Read the model definition and answer for the solid it produces. Units are mm, in the model's axes. A direction names the side the tool comes from. Give positions to 0.01 mm unless a question says otherwise; leave off trailing zeros. Order: outer loops, then holes, each group sorted by start corner. A loop starts at its lowest first (then second) coordinate and runs counter-clockwise, first axis right, second up. Notation, with made-up numbers: (26, 66) - (69, 66) arc R9 ccw to (69, 83) - close; hole circle Ø1 at (79, 1.25). An arc over 180 degrees is marked (long way). One line per item, written item: value. Start each with the question number.
```python
from build123d import *

# Parameters (mm, degrees)
F0_R     = 1
F1_DEPTH = 10


with BuildPart() as f1:
    # F0 (on Front) → F1 (new body)
    with BuildSketch(Plane.XZ):
        with BuildLine():
            Line((-1.562834, 8.86327), (-1.345773, 7.63226))
            ThreePointArc((-1.345773, 7.63226), (-2.005848, 7.485925), (-2.650656, 7.282618))
            Line((-2.650656, 7.282618), (-3.078181, 8.457234))
            ThreePointArc((-3.078181, 8.457234), (-3.540527, 8.860187), (-4.094507, 9.123322))
            Line((-4.094507, 9.123322), (-4.356972, 9.000933))
            ThreePointArc((-4.356972, 9.000933), (-4.51149, 8.407419), (-4.5, 7.794229))
            Line((-4.5, 7.794229), (-3.875, 6.711697))
            ThreePointArc((-3.875, 6.711697), (-4.445217, 6.348428), (-4.981604, 5.936844))
            Line((-4.981604, 5.936844), (-5.785088, 6.8944))
            ThreePointArc((-5.785088, 6.8944), (-6.357369, 7.114921), (-6.967938, 7.172715))
            Line((-6.967938, 7.172715), (-7.172715, 6.967938))
            ThreePointArc((-7.172715, 6.967938), (-7.114921, 6.357369), (-6.8944, 5.785088))
            Line((-6.8944, 5.785088), (-5.936844, 4.981604))
            ThreePointArc((-5.936844, 4.981604), (-6.348428, 4.445217), (-6.711697, 3.875))
            Line((-6.711697, 3.875), (-7.794229, 4.5))
            ThreePointArc((-7.794229, 4.5), (-8.407419, 4.51149), (-9.000933, 4.356972))
            Line((-9.000933, 4.356972), (-9.123322, 4.094507))
            ThreePointArc((-9.123322, 4.094507), (-8.860187, 3.540527), (-8.457234, 3.078181))
            Line((-8.457234, 3.078181), (-7.282618, 2.650656))
            ThreePointArc((-7.282618, 2.650656), (-7.485925, 2.005848), (-7.63226, 1.345773))
            Line((-7.63226, 1.345773), (-8.86327, 1.562834))
            ThreePointArc((-8.86327, 1.562834), (-9.44341, 1.363908), (-9.948283, 1.015714))
            Line((-9.948283, 1.015714), (-9.973523, 0.727218))
            ThreePointArc((-9.973523, 0.727218), (-9.536784, 0.296644), (-9, 0))
            Line((-9, 0), (-7.75, 0))
            ThreePointArc((-7.75, 0), (-7.720509, -0.675457), (-7.63226, -1.345773))
            Line((-7.63226, -1.345773), (-8.86327, -1.562834))
            ThreePointArc((-8.86327, -1.562834), (-9.340387, -1.948183), (-9.695722, -2.448054))
            Line((-9.695722, -2.448054), (-9.620769, -2.727784))
            ThreePointArc((-9.620769, -2.727784), (-9.063104, -2.983018), (-8.457234, -3.078181))
            Line((-8.457234, -3.078181), (-7.282618, -2.650656))
            ThreePointArc((-7.282618, -2.650656), (-7.023885, -3.275292), (-6.711697, -3.875))
            Line((-6.711697, -3.875), (-7.794229, -4.5))
            ThreePointArc((-7.794229, -4.5), (-8.110775, -5.025293), (-8.273715, -5.616551))
            Line((-8.273715, -5.616551), (-8.107608, -5.853776))
            ThreePointArc((-8.107608, -5.853776), (-7.496279, -5.902884), (-6.8944, -5.785088))
            Line((-6.8944, -5.785088), (-5.936844, -4.981604))
            ThreePointArc((-5.936844, -4.981604), (-5.480078, -5.480078), (-4.981604, -5.936844))
            Line((-4.981604, -5.936844), (-5.785088, -6.8944))
            ThreePointArc((-5.785088, -6.8944), (-5.902884, -7.496279), (-5.853776, -8.107608))
            Line((-5.853776, -8.107608), (-5.616551, -8.273715))
            ThreePointArc((-5.616551, -8.273715), (-5.025293, -8.110775), (-4.5, -7.794229))
            Line((-4.5, -7.794229), (-3.875, -6.711697))
            ThreePointArc((-3.875, -6.711697), (-3.275292, -7.023885), (-2.650656, -7.282618))
            Line((-2.650656, -7.282618), (-3.078181, -8.457234))
            ThreePointArc((-3.078181, -8.457234), (-2.983018, -9.063104), (-2.727784, -9.620769))
            Line((-2.727784, -9.620769), (-2.448054, -9.695722))
            ThreePointArc((-2.448054, -9.695722), (-1.948183, -9.340387), (-1.562834, -8.86327))
            Line((-1.562834, -8.86327), (-1.345773, -7.63226))
            ThreePointArc((-1.345773, -7.63226), (-0.675457, -7.720509), (0, -7.75))
            Line((0, -7.75), (0, -9))
            ThreePointArc((0, -9), (0.296644, -9.536784), (0.727218, -9.973523))
            Line((0.727218, -9.973523), (1.015714, -9.948283))
            ThreePointArc((1.015714, -9.948283), (1.363908, -9.44341), (1.562834, -8.86327))
            Line((1.562834, -8.86327), (1.345773, -7.63226))
            ThreePointArc((1.345773, -7.63226), (2.005848, -7.485925), (2.650656, -7.282618))
            Line((2.650656, -7.282618), (3.078181, -8.457234))
            ThreePointArc((3.078181, -8.457234), (3.540527, -8.860187), (4.094507, -9.123322))
            Line((4.094507, -9.123322), (4.356972, -9.000933))
            ThreePointArc((4.356972, -9.000933), (4.51149, -8.407419), (4.5, -7.794229))
            Line((4.5, -7.794229), (3.875, -6.711697))
            ThreePointArc((3.875, -6.711697), (4.445217, -6.348428), (4.981604, -5.936844))
            Line((4.981604, -5.936844), (5.785088, -6.8944))
            ThreePointArc((5.785088, -6.8944), (6.357369, -7.114921), (6.967938, -7.172715))
            Line((6.967938, -7.172715), (7.172715, -6.967938))
            ThreePointArc((7.172715, -6.967938), (7.114921, -6.357369), (6.8944, -5.785088))
            Line((6.8944, -5.785088), (5.936844, -4.981604))
            ThreePointArc((5.936844, -4.981604), (6.348428, -4.445217), (6.711697, -3.875))
            Line((6.711697, -3.875), (7.794229, -4.5))
            ThreePointArc((7.794229, -4.5), (8.407419, -4.51149), (9.000933, -4.356972))
            Line((9.000933, -4.356972), (9.123322, -4.094507))
            ThreePointArc((9.123322, -4.094507), (8.860187, -3.540527), (8.457234, -3.078181))
            Line((8.457234, -3.078181), (7.282618, -2.650656))
            ThreePointArc((7.282618, -2.650656), (7.485925, -2.005848), (7.63226, -1.345773))
            Line((7.63226, -1.345773), (8.86327, -1.562834))
            ThreePointArc((8.86327, -1.562834), (9.44341, -1.363908), (9.948283, -1.015714))
            Line((9.948283, -1.015714), (9.973523, -0.727218))
            ThreePointArc((9.973523, -0.727218), (9.536784, -0.296644), (9, 0))
            Line((9, 0), (7.75, 0))
            ThreePointArc((7.75, 0), (7.720509, 0.675457), (7.63226, 1.345773))
            Line((7.63226, 1.345773), (8.86327, 1.562834))
            ThreePointArc((8.86327, 1.562834), (9.340387, 1.948183), (9.695722, 2.448054))
            Line((9.695722, 2.448054), (9.620769, 2.727784))
            ThreePointArc((9.620769, 2.727784), (9.063104, 2.983018), (8.457234, 3.078181))
            Line((8.457234, 3.078181), (7.282618, 2.650656))
            ThreePointArc((7.282618, 2.650656), (7.023885, 3.275292), (6.711697, 3.875))
            Line((6.711697, 3.875), (7.794229, 4.5))
            ThreePointArc((7.794229, 4.5), (8.110775, 5.025293), (8.273715, 5.616551))
            Line((8.273715, 5.616551), (8.107608, 5.853776))
            ThreePointArc((8.107608, 5.853776), (7.496279, 5.902884), (6.8944, 5.785088))
            Line((6.8944, 5.785088), (5.936844, 4.981604))
            ThreePointArc((5.936844, 4.981604), (5.480078, 5.480078), (4.981604, 5.936844))
            Line((4.981604, 5.936844), (5.785088, 6.8944))
            ThreePointArc((5.785088, 6.8944), (5.902884, 7.496279), (5.853776, 8.107608))
            Line((5.853776, 8.107608), (5.616551, 8.273715))
            ThreePointArc((5.616551, 8.273715), (5.025293, 8.110775), (4.5, 7.794229))
            Line((4.5, 7.794229), (3.875, 6.711697))
            ThreePointArc((3.875, 6.711697), (3.275292, 7.023885), (2.650656, 7.282618))
            Line((2.650656, 7.282618), (3.078181, 8.457234))
            ThreePointArc((3.078181, 8.457234), (2.983018, 9.063104), (2.727784, 9.620769))
            Line((2.727784, 9.620769), (2.448054, 9.695722))
            ThreePointArc((2.448054, 9.695722), (1.948183, 9.340387), (1.562834, 8.86327))
            Line((1.562834, 8.86327), (1.345773, 7.63226))
            ThreePointArc((1.345773, 7.63226), (0.675457, 7.720509), (0, 7.75))
            Line((0, 7.75), (0, 9))
            ThreePointArc((0, 9), (-0.296644, 9.536784), (-0.727218, 9.973523))
            Line((-0.727218, 9.973523), (-1.015714, 9.948283))
            ThreePointArc((-1.015714, 9.948283), (-1.363908, 9.44341), (-1.562834, 8.86327))
        make_face()
        Circle(F0_R, mode=Mode.SUBTRACT)
    extrude(amount=F1_DEPTH)


solid = f1.part
```
1) Find the intervals of material crossed by probe 1 along X at (y, z) = (-7.25, -7); probe 2 along Z at (x, y) = (1.75, -7); probe 3 along Z at (x, y) = (-5.5, -1.75), in increasing order. Write a range as from..to.
2) For faces 1 (the cylindrical face through (1.954, -4.93, 9.346)), 2 (the cylindrical face through (-7, -5, 6)), 3 (the flat face through (8.239, -4.93, -1.453)), 4 (the cylindrical face through (0.29, -4.93, -9.53)), determine the directions among +Z, -Z, +X, -X, +Y, -Y from which every point of the face is accessible in a straight line to the end or side of a thin tool.
3) The mould has two halves that part along X. Classify faces 5 (the cylindrical face through (9.436, -4.93, -1.368)), 6 (the cylindrical face through (-8.865, -4.93, 3.548)), 7 (the cylindrical face through (3.28, -4.93, 7.02)): +X half, -X half, draft (parallel to the pull), parting line (faces both ways), or undercut.
4) Each of these flat-tipped pins is pushed along its axis until it touches: pin 1 (1.4 mm diameter, centred on y = -3.5, z = -8, fed in from -X); pin 2 (3 mm diameter, centred on y = -9, z = 6.5, fed in from -X); pin 3 (1 mm diameter, centred on x = 8.5, y = -7, fed in from +Z). Where does it stop, or does it pass through?
5) Section A-A on z = 2 is taken. Write down the section's boundary in (x, y), plus the area to 3 significant figures.
6) Section B-B on x = -2 is taken. Write down the section's boundary in (y, z).
Solved:
1. probe 1: x = -5.82..-4.04, -3.33..4.04, 6..7.14
1. probe 2: z = -7.55..9.13
1. probe 3: z = -8.26..-6.55, -5.46..6.55
2. face 1: +Z, +Y, -Y
2. face 2: -X, +Y, -Y
2. face 3: +Y, -Y
2. face 4: -Z, +Y, -Y
3. face 5: +X half
3. face 6: -X half
3. face 7: undercut
4. pin 1: stops at x = -5.91
4. pin 2: stops at x = -7.17
4. pin 3: stops at z = 5.87
5. outline: (-7.49, -10) - (9.39, -10) - (9.39, 0) - (-7.49, 0) - close
5. area: 169 mm2
6. outline: (-10, -9.39) - (0, -9.39) - (0, 7.49) - (-10, 7.49) - close
